Input: dimensioned drawing with shaded views. Units: mm. Origin: part minimum x, y, z. A direction names the side the tool comes from. Give positions to 0.01 mm unless a question says otherwise; leave off trailing zeros. Write each loop counter-clockwise with the first axis right and the second up, starting at its lowest first coordinate (ties: lowest second). Pieces come first, ordered by that corner, then holes. Notation, with made-up numbers: (42, -36.5) -> (94, -36.5) arc R25 ccw to (94, -16.5) -> close; hole circle Ø5 at (68, -36.75). An arc over 180 degrees is marked (long way). Answer in a Markdown table with one row per item. Add a question column.
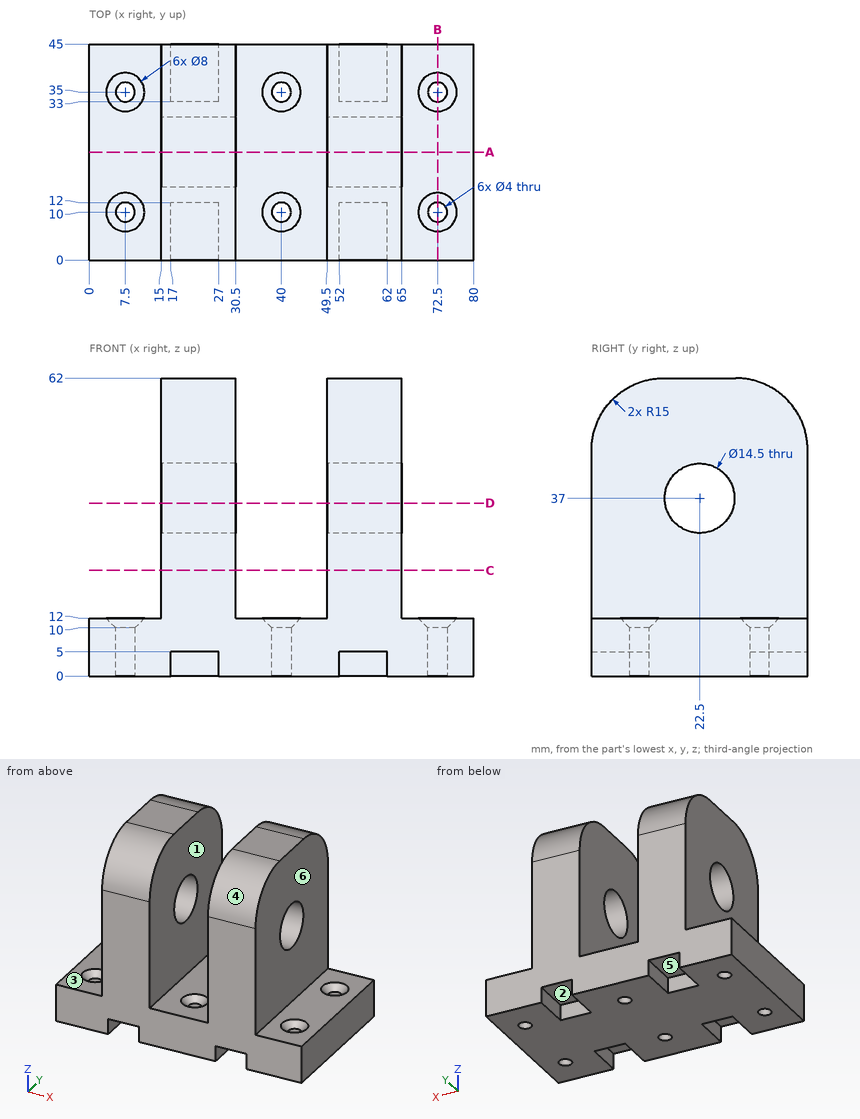
Q1. Line query: probe 1 along Y at (x, z) = (72.5, 7.25); probe 2 along X at (y, z) = (43.5, 45); probe 3 along Y at (x, z) = (40.5, 3.5). Output: solid intervals per line, ascending. Write a range as from..to.
Q2. Contact query for flat-ended pins moving along their axis: pin 1 Ø1 at (y, z) = (9, 34) entering from -X; pin 2 Ø4 at (x, z) = (13.5, 55) entering from +Y; pin 3 Ø2.5 at (x, z) = (59, 3.5) entering from -Y; pin 4 Ø2.5 at (x, y) = (40, 10) entering from +Z. Output: stop coordinate, or through.
Q3. Section C-C on z = 22. Return loops of the section in (x, y), and give its area (4 significant figures).
Q4. Access query for the marked faces 1, 2 and 3. Directions: +Z, -Z, +X, -X, +Y, -Y. A direction counts if a zero-diameter tool reaches every point of the face in a straight line with its end or side. Return the directions, or none.
Q5. Section A-A on y = 22.5. Return loops of the section in (x, z), and give its area (3 significant figures).
Q6. Section D-D on z = 36. Return loops of the section in (x, y).
Q7. Section B-B on x = 72.5. Return loops of the section in (y, z), and give its area (3 significant figures).
Q8. Pull-direction query (X, two-part tool) for the marked faces 4, 5 and 6; classes: +X half, -X half, draft (parallel to the pull), parting line (faces both ways), or undercut.
Checks:
| question | item | result |
|---|---|---|
| 1 | probe 1 | 0..8, 12..33, 37..45 |
| 1 | probe 2 | 15..30.5, 49.5..65 |
| 1 | probe 3 | 0..8.06, 11.94..33.06, 36.94..45 |
| 2 | pin 1 | x = 15 |
| 2 | pin 2 | y = 43.43 |
| 2 | pin 3 | y = 12 |
| 2 | pin 4 | through |
| 3 | outline | (15, 0) -> (30.5, 0) -> (30.5, 45) -> (15, 45) -> close; (49.5, 0) -> (65, 0) -> (65, 45) -> (49.5, 45) -> close |
| 3 | area | 1,395 mm^2 |
| 4 | face 1 | +Z, +Y, -Y |
| 4 | face 2 | -Z, +Y |
| 4 | face 3 | +Z, -X, +Y, -Y |
| 5 | outline | (0, 0) -> (80, 0) -> (80, 12) -> (65, 12) -> (65, 29.75) -> (49.5, 29.75) -> (49.5, 12) -> (30.5, 12) -> (30.5, 29.75) -> (15, 29.75) -> (15, 12) -> (0, 12) -> close; (15, 44.25) -> (30.5, 44.25) -> (30.5, 62) -> (15, 62) -> close; (49.5, 44.25) -> (65, 44.25) -> (65, 62) -> (49.5, 62) -> close |
| 5 | area | 2,060 mm^2 |
| 6 | outline | (15, 0) -> (30.5, 0) -> (30.5, 15.32) -> (15, 15.32) -> close; (15, 29.68) -> (30.5, 29.68) -> (30.5, 45) -> (15, 45) -> close; (49.5, 0) -> (65, 0) -> (65, 15.32) -> (49.5, 15.32) -> close; (49.5, 29.68) -> (65, 29.68) -> (65, 45) -> (49.5, 45) -> close |
| 7 | outline | (0, 0) -> (8, 0) -> (8, 10) -> (6, 12) -> (0, 12) -> close; (12, 0) -> (33, 0) -> (33, 10) -> (31, 12) -> (14, 12) -> (12, 10) -> close; (37, 0) -> (45, 0) -> (45, 12) -> (39, 12) -> (37, 10) -> close |
| 7 | area | 436 mm^2 |
| 8 | face 4 | draft |
| 8 | face 5 | undercut |
| 8 | face 6 | +X half |
